```python
from build123d import *

# Parameters (mm, degrees)
F0_R     = 1
F1_DEPTH = 100


with BuildPart() as f1:
    # F0 (on Front) → F1 (new body)
    with BuildSketch(Plane.XZ):
        Circle(F0_R)
    extrude(amount=F1_DEPTH)

    # F2 (on face) → F3 (revolve)
    with BuildSketch(Plane.XZ.offset(100)):
        with BuildLine():
            Line((0, 1), (0, 5))
            ThreePointArc((0, 5), (-5, 0), (0, -5))
            Line((0, -5), (0, -1))
            ThreePointArc((0, -1), (-1, 0), (0, 1))
        make_face()
    revolve(axis=Axis((0, -100, 0), (0, 0, -1)))

    # F4: F1 across plane


with BuildPart() as f1_1:
    add(f1.part)
    add(f1.part.mirror(Plane.XZ))


solid = f1_1.part
```
Design review of the part built by this model. Coordinates are the model's own, in mm. Coordinates: 2 decimals unless noted, no trailing zeros. Order: outer loops, then holes, each group sorted by start corner. A loop starts at its lowest first (then second) coordinate and runs counter-clockwise, first axis right, second up.
1) Take a section at B-B, the plane y = 13. Give the boundary of the cut face in (x, z).
2) Take a section at A-A, the plane x = 2.75. Give the boundary of the cut face in (y, z).
3) Clearance check with flat-ended pins moving along their axes: pin 1 (4 mm diameter, centred on x = 1, z = -4, fed in from -Y); pin 2 (4 mm diameter, centred on x = 2.5, y = 64.5, fed in from -Z); pin 3 (4 mm diameter, centred on y = 33.5, z = 2, fed in from +X); pin 4 (2 mm diameter, centred on x = 0.5, z = -0.5, fed in from -Y). State where each tip first meets the part, or that it passes through.
4) Wall thickness on line 1 along Y through (x, z) = (-1.5, 2.5); line 2 along X through (y, z) = (-83.5, 0.25); line 3 along Y through (x, z) = (3.75, -1): over which ranges is each line inside the solid? List them lowest first.
Returned:
1. outline: circle Ø2 at (0, 0)
2. outline: circle Ø8.35 at (-100, 0); circle Ø8.35 at (100, 0)
3. pin 1: stops at y = -104.53
3. pin 2: stops at z = -0.87
3. pin 3: stops at x = 1
3. pin 4: stops at y = -105
4. line 1: y = -104.06 to -95.94, 95.94 to 104.06
4. line 2: x = -0.97 to 0.97
4. line 3: y = -103.15 to -96.85, 96.85 to 103.15
